Source: CAD feature listing. Evaluate the final solid. Frame: model axes, mm. A direction names the side the tool comes from. Round coordinates to 2 decimals unless told otherwise and drop trailing zeros. Order: outer loops, then holes, each group sorted by start corner. A loop starts at its lowest first (then second) coordinate and runs counter-clockwise, first axis right, second up. Notation, with made-up numbers: (55, 72.25) -> (102, 72.25) arc R17 cw to (102, 78.25) -> close; hole circle Ø9 at (23, 30.25). An arc over 180 degrees is marked (long way). Answer as CSV lines item,"result". Start each with the question number.
(1) Contact query for flat-ended pins moving along their axis: P1, Ø1.5, axis at x = 8, z = -73.5, coming from the -Y side; P2, Ø3, axis at x = 7.5, z = -22, coming from the -Y side; P3, Ø6, axis at x = 9.5, z = -19.5, coming from the +Y side; P4, Ø5, axis at y = 28.5, z = -68.5, coming from the -X side. Output: stop coordinate, or through.
(2) Set-up query: faces 5 (the flat face through (9, 28, -20)), 6 (the flat face through (18, 0, -59)), 7 (the flat face through (9, 28, -59)). Return all of +Z, -Z, +X, -X, +Y, -Y with unobstructed straight access to the full face (end or side cutting, diameter ignored); none if empty.
(3) Section query C-C (y = 8). Output: boundary loops of the cut face in (x, z), plus the area to 3 significant figures.
(4) Line query: line 1 along X through (y, z) = (29.5, -72.5); line 2 along Y through (x, z) = (19, -58.5); line 3 along Z through (x, y) = (24, 54). Output: solid intervals per line, ascending. Write a range as from..to.
(5) Section query D-D (z = -60). Output: boundary loops of the cut face in (x, y).
(6) Section query A-A (z = -7.5). Output: boundary loops of the cut face in (x, y), plus the area to 4 significant figures.
(7) Pull-direction query (Y, two-part tool) for faces 1 (the flat face through (18, 65, -57)), 2 (the flat face through (18, 57, -61.619)), 3 (the flat face through (6.5, 28, -10)), 4 (the flat face through (17.75, 7.6, -1.48)); classes: +Y half, -Y half, draft (parallel to the pull), parting line (faces both ways), or undercut.
(8) Section query B-B (x = 22.5). Output: boundary loops of the cut face in (y, z) (3 decimals).
```python
from build123d import *

# Parameters (mm, degrees)
EXTRUDE_1_DEPTH     = 36
SKETCH_2_W          = 5
SKETCH_2_H          = 6.5
CUT_EXTRUDE_1_DEPTH = 20
SKETCH_3_W          = 5
SKETCH_3_H          = 6.5
CUT_EXTRUDE_2_DEPTH = 20


with BuildPart() as part:
    # Эскиз1 → Бобышка-Вытянуть1 (new body)
    with BuildSketch(Plane(origin=(0, 0, 0), x_dir=(0, 0, -1), z_dir=(1, 0, 0))):
        with BuildLine():
            Line((0, 15), (3, 0))
            Line((3, 0), (20, 0))
            Line((20, 0), (21.5, 1.565195477))
            Line((21.5, 1.565195477), (21.5, 5))
            Line((21.5, 5), (57.5, 5))
            Line((57.5, 5), (57.5, 3))
            Line((57.5, 3), (55.5, 0))
            Line((55.5, 0), (62, 0))
            Line((62, 0), (79, 4))
            Line((79, 4), (79, 50))
            Line((79, 50), (61.619424271, 50))
            Line((61.619424271, 50), (61.619424271, 65))
            Line((61.619424271, 65), (52.96803048, 65))
            ThreePointArc((52.96803048, 65), (48.430063355, 67.893872917), (43.892096231, 65))
            Line((43.892096231, 65), (42.98652577, 67))
            Line((42.98652577, 67), (22.355935477, 65))
            Line((22.355935477, 65), (17, 65))
            Line((17, 65), (17, 50))
            Line((17, 50), (0, 50))
            Line((0, 50), (0, 15))
        make_face()
    extrude(amount=EXTRUDE_1_DEPTH)

    # Эскиз2 → Вырез-Вытянуть1 (cut)
    with BuildSketch(Plane(origin=(0, 0, -79), x_dir=(-1, 0, 0), z_dir=(0, 0, -1))):
        with Locations((-27, 28.25)):
            Rectangle(SKETCH_2_W, SKETCH_2_H)
        with Locations((-9, 28.25)):
            Rectangle(SKETCH_2_W, SKETCH_2_H)
    extrude(amount=-CUT_EXTRUDE_1_DEPTH, mode=Mode.SUBTRACT)

    # Эскиз3 → Вырез-Вытянуть2 (cut)
    with BuildSketch(Plane.XY):
        with Locations((9, 28.25)):
            Rectangle(SKETCH_3_W, SKETCH_3_H)
        with Locations((27, 28.25)):
            Rectangle(SKETCH_3_W, SKETCH_3_H)
    extrude(amount=-CUT_EXTRUDE_2_DEPTH, mode=Mode.SUBTRACT)


solid = part.part
```
Answer block:
1,P1,"y = 2.53"
1,P2,"y = 0.52"
1,P3,"y = 65.01"
1,P4,"x = 0"
2,face 5,"+Z"
2,face 6,"+Z, -Z, +X, -X, -Y"
2,face 7,"-Z"
3,outline,"(0, -79) -> (36, -79) -> (36, -1.4) -> (0, -1.4) -> close"
3,area,"2,790 mm2"
4,line 1,"0..6.5, 11.5..24.5, 29.5..36"
4,line 2,"0..65"
4,line 3,"-61.62..-17"
5,outline,"(0, 0) -> (36, 0) -> (36, 65) -> (0, 65) -> close; hole (6.5, 25) -> (11.5, 25) -> (11.5, 31.5) -> (6.5, 31.5) -> close; hole (24.5, 25) -> (29.5, 25) -> (29.5, 31.5) -> (24.5, 31.5) -> close"
6,outline,"(0, 0) -> (36, 0) -> (36, 50) -> (0, 50) -> close; hole (6.5, 25) -> (11.5, 25) -> (11.5, 31.5) -> (6.5, 31.5) -> close; hole (24.5, 25) -> (29.5, 25) -> (29.5, 31.5) -> (24.5, 31.5) -> close"
6,area,"1,735 mm2"
7,face 1,"+Y half"
7,face 2,"draft"
7,face 3,"undercut"
7,face 4,"-Y half"
8,outline,"(0, -62) -> (4, -79) -> (50, -79) -> (50, -61.619) -> (65, -61.619) -> (65, -52.968) arc R5.005 ccw to (65, -43.892) -> (67, -42.987) -> (65, -22.356) -> (65, -17) -> (50, -17) -> (50, 0) -> (15, 0) -> (0, -3) -> (0, -20) -> (1.565, -21.5) -> (5, -21.5) -> (5, -57.5) -> (3, -57.5) -> (0, -55.5) -> close"
